```python
from build123d import *

# Parameters (mm, degrees)
SKETCH1_R           = 13
SKETCH1_R_2         = 1.5
BOSS_EXTRUDE1_DEPTH = 3


with BuildPart() as part:
    # Sketch1 → Boss-Extrude1 (new body)
    with BuildSketch(Plane(origin=(0, 0, 0), x_dir=(1, 0, 0), z_dir=(0, 1, 0))):
        Circle(SKETCH1_R)
        with Locations((-2.588190451, -9.659258263)):
            Circle(SKETCH1_R_2, mode=Mode.SUBTRACT)
        with Locations((2.588190451, 9.659258263)):
            Circle(SKETCH1_R_2, mode=Mode.SUBTRACT)
        with BuildLine():
            Line((-3.059411708, 1.7), (3.059411708, 1.7))
            ThreePointArc((3.059411708, 1.7), (3.5, 0), (3.059411708, -1.7))
            Line((3.059411708, -1.7), (-3.059411708, -1.7))
            ThreePointArc((-3.059411708, -1.7), (-3.5, 0), (-3.059411708, 1.7))
        make_face(mode=Mode.SUBTRACT)
    extrude(amount=BOSS_EXTRUDE1_DEPTH)


solid = part.part
```
Here's how the part is built. I have some questions about the finished solid (model axes, mm). A direction names the side the tool comes from. Coordinates: 2 decimals unless noted, no trailing zeros. Order: outer loops, then holes, each group sorted by start corner. A loop starts at its lowest first (then second) coordinate and runs counter-clockwise, first axis right, second up. Notation, with made-up numbers: (88.5, 83) - (141.5, 83) arc R10 ccw to (141.5, 101) - close; hole circle Ø10 at (-24.75, 57.25). An arc over 180 degrees is marked (long way). One line per question, with ' | ' between items. Start each with the question number.
1. If we mould it in two halves opening along X, with no side actions, what happens to faces 1 (the cylindrical face through (-10.316, 1.479, 7.91)), 2 (the flat face through (0, 0, 3)), 3 (the flat face through (0, 1, 1.7))? For each: released by +X, released by -X, zero draft, split by the parting line, or undercut.
2. I'm going to push flat-ended pins straight in: pin 1 Ø1.8 at (x, z) = (2.59, -9.66) entering from +Y; pin 2 Ø1 at (x, y) = (2.5, 2) entering from +Z. Where does each tip first touch, or does it pass through?
3. If we section it at A-A (x = 0): Write out the boundary of the cut face in (y, z).
4. If we section it at C-C (y = 2.6): Write out the boundary of the cut face in (x, z).
5. Please list where these lines run through material, in increasing order: line 1 along Z through (x, y) = (0, 1.7); line 2 along Z through (x, y) = (-2, 2.55); line 3 along Z through (x, y) = (3, 1.25). Write a range as [from, to].
6. If we section it at D-D (x = 4.5): Write out the boundary of the cut face in (y, z).
7. Which directions (+Z, -Z, +X, -X, +Y, -Y) give clear straight access to the entire face, cutting with the end or side of a thin tool? Please do faces 4 (the flat face through (0, 3, 3)), 5 (the cylindrical face through (3.5, 1.5, 0)).
8. If we section it at B-B (z = 0): Write out the boundary of the cut face in (x, y).
Model answer:
1) face 1: split by the parting line | face 2: zero draft | face 3: undercut
2) pin 1: passes through | pin 2: stops at z = 12.85
3) outline: (0, -13) - (3, -13) - (3, -1.7) - (0, -1.7) - close; (0, 1.7) - (3, 1.7) - (3, 13) - (0, 13) - close
4) outline: circle Ø26 at (0, 0); hole circle Ø3 at (-2.59, 9.66); hole (-3.06, -1.7) - (3.06, -1.7) arc R3.5 ccw to (3.06, 1.7) - (-3.06, 1.7) arc R3.5 ccw to start; hole circle Ø3 at (2.59, -9.66)
5) line 1: z = [-13, -1.7], [1.7, 13] | line 2: z = [-12.85, -1.7], [1.7, 8.28], [11.04, 12.85] | line 3: z = [-12.65, -11.1], [-8.22, -1.7], [1.7, 12.65]
6) outline: (0, -12.2) - (3, -12.2) - (3, 12.2) - (0, 12.2) - close
7) face 4: +Z, -Z, +X, -X, +Y | face 5: +Y, -Y
8) outline: (-13, 0) - (-3.5, 0) - (-3.5, 3) - (-13, 3) - close; (3.5, 0) - (13, 0) - (13, 3) - (3.5, 3) - close
